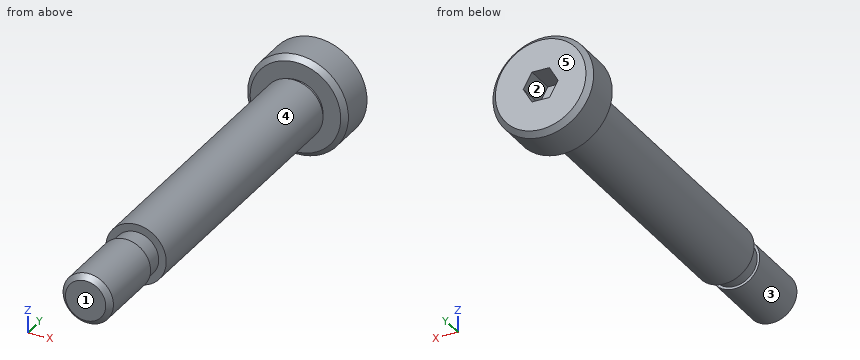
from build123d import *

# Parameters (mm, degrees)
CHAMFER1_SIZE      = 0.5
CUT_EXTRUDE1_DEPTH = 3


with BuildPart() as part:
    # Sketch1 → Revolve1 (revolve)
    with BuildSketch(Plane.XY, mode=Mode.PRIVATE) as revolve1_sk:
        Polygon((0, 0), (5, 0), (5, -4.5), (2.75, -4.5), (2.75, -5), (3, -5), (3, -34.5), (2.25, -34.5), (2.25, -36.5), (2.5, -36.5), (2.5, -44), (0, -44), align=None)
    revolve(revolve1_sk.sketch.rotate(Axis((0, 3, 0), (0, -1, 0)), 180), axis=Axis((0, 3, 0), (0, -1, 0)))

    # Chamfer1
    chamfer1_edges = [part.edges().sort_by_distance(p)[0] for p in [
        (5, -4.5, 0),
        (5, 0, 0),
        (2.5, -44, 0),
    ]]
    chamfer(chamfer1_edges, length=CHAMFER1_SIZE)

    # Sketch2 → Cut-Extrude1 (cut)
    with BuildSketch(Plane(origin=(0, 0, 0), x_dir=(1, 0, 0), z_dir=(0, 1, 0))):
        Polygon((1.732050808, 0), (0.866025404, 1.5), (-0.866025404, 1.5), (-1.732050808, 0), (-0.866025404, -1.5), (0.866025404, -1.5), align=None)
    extrude(amount=-CUT_EXTRUDE1_DEPTH, mode=Mode.SUBTRACT)


solid = part.part
Check sheet for the modelled part. Datum: model origin and axes. Units: mm. Face numbers are marked on the shaded views. A direction names the side the tool comes from. Round coordinates to 2 decimals unless told otherwise and drop trailing zeros. Loops run counter-clockwise (first coordinate to the right, second up) from the corner with the lowest first, then second, coordinate; pieces in that order, holes last. Notation, with made-up numbers: M 37,-9.5 L 49,-9.5 A35 ccw 49,26.5 Z; hole C -10,-17 d7. An arc over 180 degrees is marked long. One line per question, with ' | ' between items. Start each with the question number.
Item 1: Section check D-D (y = -16). Record the boundary of the cut face in (x, z), and give its area (3 significant figures).
Item 2: Section check A-A (y = -2.5). Record the boundary of the cut face in (x, z), and give its area (3 significant figures).
Item 3: Scan lines: probe 1 along Y at (x, z) = (-2, -2); probe 2 along Y at (x, z) = (1, 0.25); probe 3 along X at (y, z) = (-40.5, 2). Record each from-to range of solid material in increasing order.
Item 4: Gauge pin test, flat ends, axial feed: pin 1 Ø0.9 at (x, z) = (0, -0.5) entering from +Y; pin 2 Ø0.5 at (x, y) = (0.5, -1.5) entering from +Z; pin 3 Ø5 at (x, y) = (2, -21) entering from +Z. Record the tip position at first contact, or that the pin passes through.
Item 5: Release check for a two-part mould opening along X. For the marked faces 1, 2 and 3 record: released by +X, released by -X, zero draft, split by the parting line, or undercut.
Item 6: Section check C-C (y = -38.5). Record the boundary of the cut face in (x, z), and give its area (3 significant figures).
Item 7: Set-up check for the marked faces 4 and 5: record each of +Z, -Z, +X, -X, +Y, -Y from which the full face is reachable in a straight line by a thin tool's end or side.
Worked out:
1) outline: C 0,0 d6 | area: 28.3 mm^2
2) outline: C 0,0 d10; hole M -1.73,0 L -0.87,-1.5 L 0.87,-1.5 L 1.73,0 L 0.87,1.5 L -0.87,1.5 Z | area: 70.7 mm^2
3) probe 1: -34.5 to -5, -4.5 to 0 | probe 2: -44 to -3 | probe 3: -1.5 to 1.5
4) pin 1: y = -3 | pin 2: z = 4.99 | pin 3: z = 3
5) face 1: zero draft | face 2: undercut | face 3: split by the parting line
6) outline: C 0,0 d5 | area: 19.6 mm^2
7) face 4: -Y | face 5: +Z, -Z, +X, -X, +Y
